Can you work these out from the drawing? Everything is in mm from the part's minimum corner. Coordinates: 2 decimals unless noted, no trailing zeros. Loops run counter-clockwise (first coordinate to the right, second up) from the corner with the lowest first, then second, coordinate; pieces in that order, holes last.
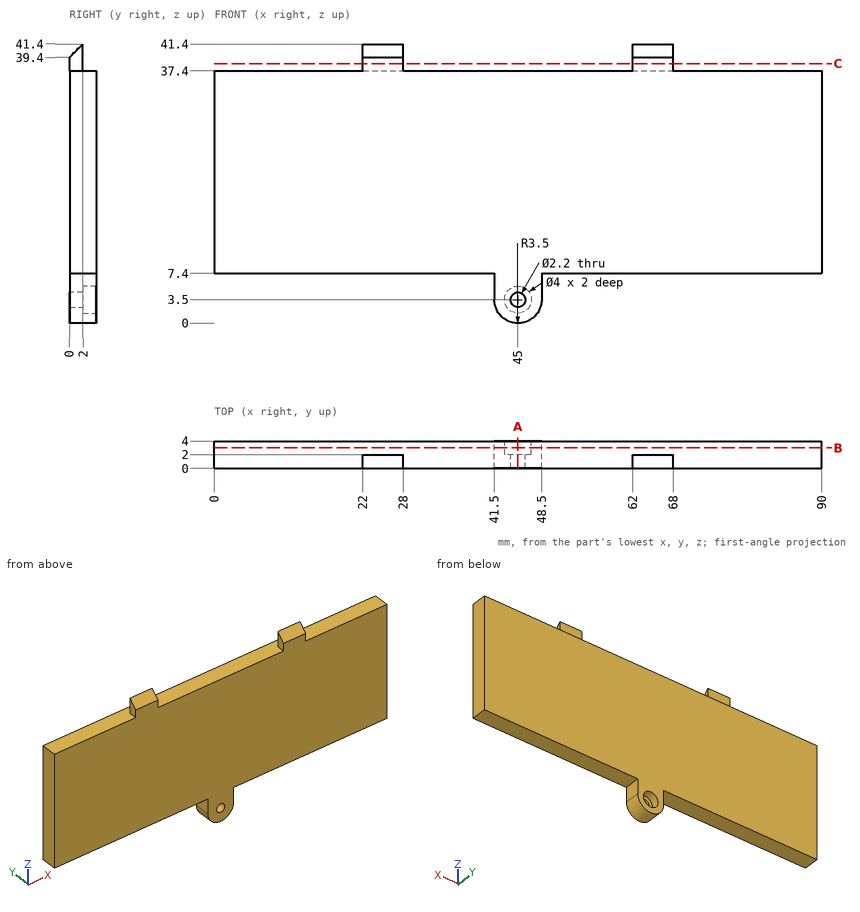
1) Imagine slicing it at B-B on y = 3. List the corners of the cut face in (x, z) for me, plus the area to 3 significant figures.
2) Will these pins go through, and if not, where does the flat tip stop? pin 1 (1.2 mm diameter, centred on x = 65.5, y = 2, fed in from -Z); pin 2 (0.6 mm diameter, centred on y = 1, z = 40, fed in from -X); pin 3 (2 mm diameter, centred on x = 25.5, y = 1.5, fed in from +Z).
3) Imagine slicing it at C-C on z = 38.5. List the corners of the cut face in (x, y) for me, plus the area to 3 significant figures.
4) If I drill on L1, parallel to X at y = 2.9, z = 3.5; L2, parallel to X at y = 0.9, z = 3.5; L3, parallel to Z at x = 75.5, y = 3.85, over which ranges is the centre line in solid material (lowest first)?
5) Imagine slicing it at A-A on x = 45. List the corners of the cut face in (y, z) for me, plus the area to 3 significant figures.
Solved:
1. outline: (0, 7.4) - (41.5, 7.4) - (41.5, 3.5) arc R3.5 ccw to (48.5, 3.5) - (48.5, 7.4) - (90, 7.4) - (90, 37.4) - (0, 37.4) - close; hole circle Ø4 at (45, 3.5)
1. area: 2,730 mm2
2. pin 1: stops at z = 7.4
2. pin 2: stops at x = 22
2. pin 3: stops at z = 41.4
3. outline: (22, 0) - (28, 0) - (28, 2) - (22, 2) - close; (62, 0) - (68, 0) - (68, 2) - (62, 2) - close
3. area: 24.0 mm2
4. L1: x = 41.5 to 43, 47 to 48.5
4. L2: x = 41.5 to 43.9, 46.1 to 48.5
4. L3: z = 7.4 to 37.4
5. outline: (0, 0) - (4, 0) - (4, 1.5) - (2, 1.5) - (2, 2.4) - (0, 2.4) - close; (0, 4.6) - (2, 4.6) - (2, 5.5) - (4, 5.5) - (4, 37.4) - (0, 37.4) - close
5. area: 137 mm2
